Geometry check sheet. Reference: drawing and pictorial views, mm from the part's lowest x, y, z. A direction names the side the tool comes from. Coordinates: 2 decimals unless noted, no trailing zeros. Loops run counter-clockwise (first coordinate to the right, second up) from the corner with the lowest first, then second, coordinate; pieces in that order, holes last. Notation, with made-up numbers: (85.5, 54) - (105.5, 54) arc R19 cw to (105.5, 59) - close; hole circle Ø8 at (4.25, 53.5). An arc over 180 degrees is marked (long way). One line per item, written item: value.
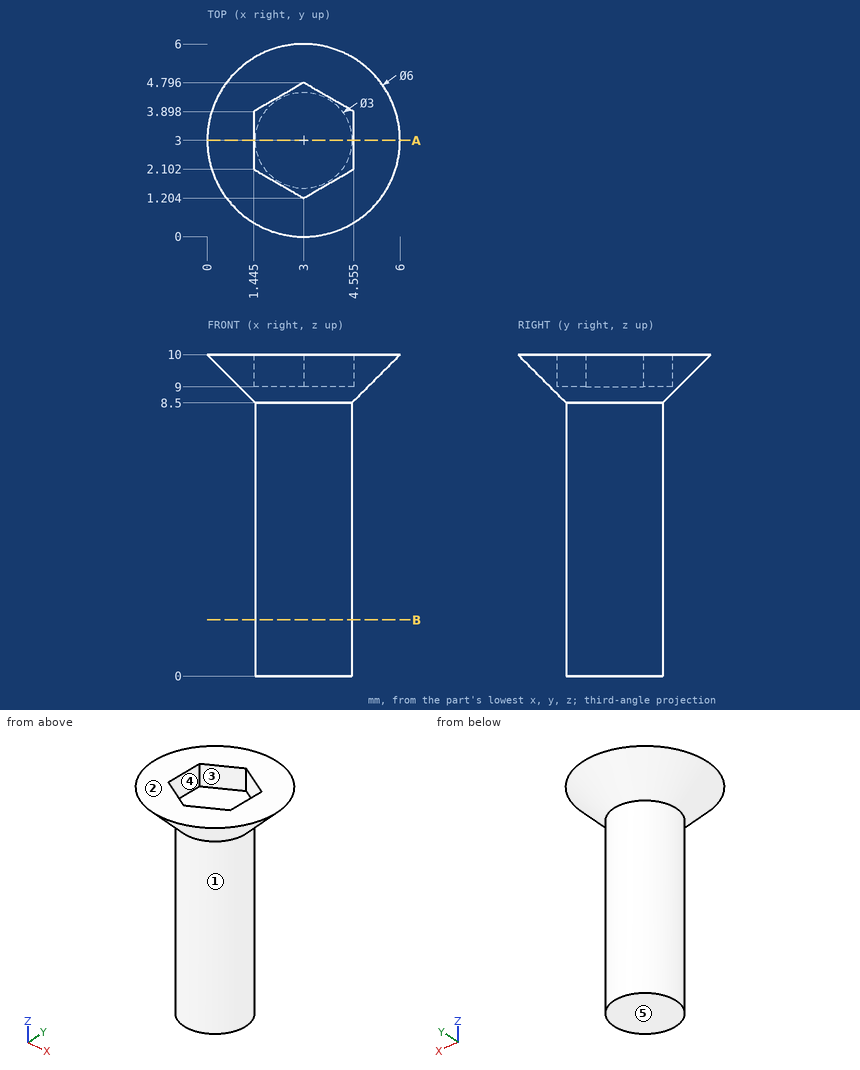
(1) Go/stop test with a flat-tipped pin: pin 1 Ø1.5 at (x, z) = (5, 5) entering from +Y. Record where the tip stops, or that it passes through.
Reply:
pin 1: y = 3.83
(2) Cross-section at A-A on y = 3. Record the cut outline in (x, z) (1 decimal).
Reply:
outline: (0, 10) - (1.5, 8.5) - (1.5, 0) - (4.5, 0) - (4.5, 8.5) - (6, 10) - (4.6, 10) - (4.6, 9) - (1.4, 9) - (1.4, 10) - close
(3) Access from +Z, -Z, +X, -X, +Y, -Y to the whole of each face (thin tool, end or side, straight path). Record for the marked faces 4 and 5.
Reply:
face 4: +Z
face 5: -Z, +X, -X, +Y, -Y
(4) Release check for a two-part mould opening along X. For the marked faces 1, 2 and 3 record: pulls with the +X half, pulls with the -X half, needs draft (parallel to the pull), parting line crosses it, or undercut.
Reply:
face 1: parting line crosses it
face 2: needs draft
face 3: undercut
(5) Material ranges on probe 1 along Z at (x, y) = (4.1, 2.7); probe 2 along X at (y, z) = (2.9, 5.25); probe 3 along Y at (x, z) = (1.8, 7.5), recorded low to high. Write a range as from..to.
Reply:
probe 1: 0..9
probe 2: 1.5..4.5
probe 3: 2.1..3.9
(6) Cross-section at B-B on z = 1.75. Record the cut outline in (x, y).
Reply:
outline: circle Ø3 at (3, 3)
